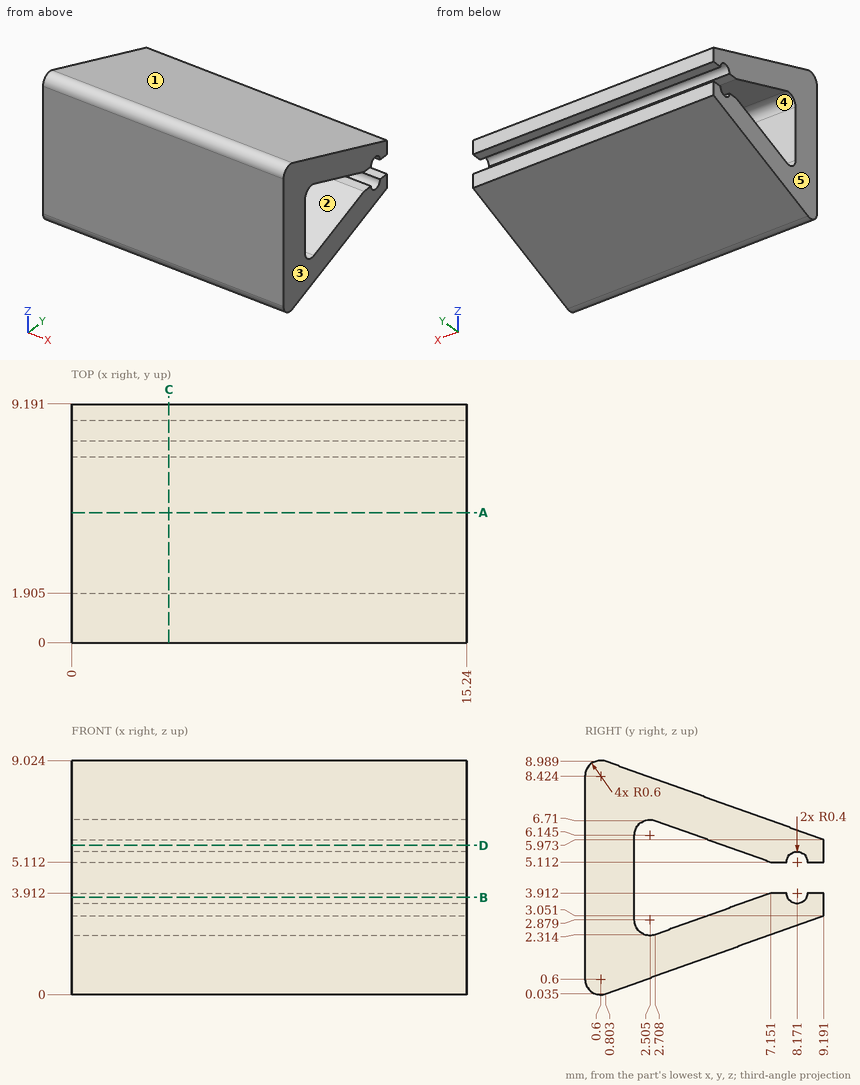
Design review of the part shown in the three views and the two pictorial views. Dimensions are in mm from the part's minimum x, y and z. A direction names the side the tool comes from. Give positions to 0.01 mm unless a question says otherwise; leave off trailing zeros. Write each loop counter-clockwise with the first axis right and the second up, starting at its lowest first coordinate (ties: lowest second). Pieces come first, ordered by that corner, then holes. Notation, with made-up numbers: M 25,-18 L 74,-18 A18 ccw 74,12 Z; hole C 49.25,39 d1. An arc over 180 degrees is marked long. Return JSON: item names as keys, results as strings. Group by question number.
Item 1: The part is to be moulded in two halves that separate along Z. For the marked faces 1, 2 and 3, say which applies: pulls with the +Z half, pulls with the -Z half, needs draft (parallel to the pull), parting line crosses it, or undercut.
Item 2: Take a section at B-B (z = 3.75). Give the boundary of the cut face in (x, y) (1 decimal).
Item 3: Take a section at D-D (z = 5.75). Give the boundary of the cut face in (x, y) (1 decimal).
Item 4: Take a section at C-C (x = 3.75). Give the boundary of the cut face in (y, z) (1 decimal).
Item 5: Tool access review of the marked faces 4 and 5: name each direction out of +Z, -Z, +X, -X, +Y, -Y from which nothing blocks a thin tool from reaching the whole face with its end or side.
Item 6: Clearance check with flat-ended pins moving along their axes: pin 1 Ø1.5 at (x, y) = (7.5, 3) entering from -Z (1 decimal); pin 2 Ø1 at (x, y) = (6.5, 2) entering from +Z; pin 3 Ø0.7 at (x, y) = (7.5, 7.5) entering from -Z. State where each tip first meets the part, or that it passes through.
Item 7: Wall thickness on line 1 along Z through (x, y) = (13.75, 4.5) (1 decimal); line 2 along Y through (x, z) = (12, 4.75) (1 decimal); line 3 along Z through (x, y) = (6, 5) (1 decimal): over which ranges is each line inside the solid? List them lowest first.
Item 8: Take a section at A-A (y = 5). Give the boundary of the cut face in (x, z) (1 decimal).
Return value:
{
 "1": {"face 1": "pulls with the +Z half", "face 2": "undercut", "face 3": "needs draft"},
 "2": {"outline": "M 0,0 L 15.2,0 L 15.2,1.9 L 0,1.9 Z; M 0,6.7 L 15.2,6.7 L 15.2,7.8 L 0,7.8 Z; M 0,8.5 L 15.2,8.5 L 15.2,9.2 L 0,9.2 Z"},
 "3": {"outline": "M 0,0 L 15.2,0 L 15.2,1.9 L 0,1.9 Z; M 0,5.4 L 15.2,5.4 L 15.2,9.2 L 0,9.2 Z"},
 "4": {"outline": "M 0,0.6 A0.6 ccw 0.8,0 L 9.2,3.1 L 9.2,3.9 L 8.6,3.9 A0.4 cw 7.8,3.9 L 7.2,3.9 L 2.7,2.3 A0.6 cw 1.9,2.9 L 1.9,6.1 A0.6 cw 2.7,6.7 L 7.2,5.1 L 7.8,5.1 A0.4 cw 8.6,5.1 L 9.2,5.1 L 9.2,6 L 0.8,9 A0.6 ccw 0,8.4 Z"},
 "5": {"face 4": "+X, -X", "face 5": "+Z, -Z, -X, +Y, -Y"},
 "6": {"pin 1": "stops at z = 0.6", "pin 2": "stops at z = 8.74", "pin 3": "stops at z = 2.32"},
 "7": {"line 1": "z = 1.4 to 3, 6.1 to 7.7", "line 2": "y = 0 to 1.9", "line 3": "z = 1.5 to 3.1, 5.9 to 7.5"},
 "8": {"outline": "M 0,1.5 L 15.2,1.5 L 15.2,3.1 L 0,3.1 Z; M 0,5.9 L 15.2,5.9 L 15.2,7.5 L 0,7.5 Z"}
}
